```python
from build123d import *

# Parameters (mm, degrees)
BOSS_EXTRUDE1_DEPTH = 6.35


with BuildPart() as part:
    # Model → Boss-Extrude1 (new body)
    with BuildSketch(Plane.XY):
        with BuildLine():
            Line((-1e-09, 914.4), (-194.479849893, 914.4))
            ThreePointArc((-194.479849893, 914.4), (-204.918872942, 907.625287079), (-202.98320057, 895.332073104))
            ThreePointArc((-202.98320057, 895.332073104), (-164.535916974, 779.903104595), (-165.892020398, 658.247026365))
            Line((-165.892020398, 658.247026365), (-165.93888619, 658.129795087))
            ThreePointArc((-165.93888619, 658.129795087), (-191.627212467, 575.297388544), (-239.683438481, 503.105305724))
            ThreePointArc((-239.683438481, 503.105305724), (-421.799875665, 296.628923535), (-582.037423101, 72.747657041))
            ThreePointArc((-582.037423101, 72.747657041), (-620.33909224, 32.211350911), (-671.307126154, 9.573561873))
            ThreePointArc((-671.307126154, 9.573561873), (-674.990888605, 5.409489793), (-676.274252254, 0))
            ThreePointArc((-676.274252254, 0), (-674.990888605, -5.409489793), (-671.307126154, -9.573561873))
            ThreePointArc((-671.307126154, -9.573561873), (-620.33909224, -32.211350911), (-582.037423101, -72.747657041))
            ThreePointArc((-582.037423101, -72.747657041), (-421.799875665, -296.628923535), (-239.683438481, -503.105305724))
            ThreePointArc((-239.683438481, -503.105305724), (-191.627212467, -575.297388544), (-165.93888619, -658.129795087))
            Line((-165.93888619, -658.129795087), (-165.892020398, -658.247026365))
            ThreePointArc((-165.892020398, -658.247026365), (-164.535916974, -779.903104595), (-202.98320057, -895.332073104))
            ThreePointArc((-202.98320057, -895.332073104), (-204.918872942, -907.625287079), (-194.479849893, -914.4))
            Line((-194.479849893, -914.4), (-1e-09, -914.4))
            Line((-1e-09, -914.4), (194.47984989, -914.4))
            ThreePointArc((194.47984989, -914.4), (204.918872939, -907.625287079), (202.983200567, -895.332073104))
            ThreePointArc((202.983200567, -895.332073104), (164.535916972, -779.903104595), (165.892020395, -658.247026365))
            Line((165.892020395, -658.247026365), (165.938886187, -658.129795086))
            ThreePointArc((165.938886187, -658.129795086), (191.627212464, -575.297388544), (239.683438478, -503.105305724))
            ThreePointArc((239.683438478, -503.105305724), (421.79987566, -296.628923537), (582.037423094, -72.747657046))
            ThreePointArc((582.037423094, -72.747657046), (620.339092235, -32.211350913), (671.307126151, -9.573561873))
            ThreePointArc((671.307126151, -9.573561873), (674.990888602, -5.409489793), (676.274252251, 0))
            ThreePointArc((676.274252251, 0), (674.990888602, 5.409489793), (671.307126151, 9.573561873))
            ThreePointArc((671.307126151, 9.573561873), (620.339092237, 32.211350911), (582.037423097, 72.747657043))
            ThreePointArc((582.037423097, 72.747657043), (421.799875662, 296.628923535), (239.683438478, 503.105305724))
            ThreePointArc((239.683438478, 503.105305724), (191.627212464, 575.297388544), (165.938886187, 658.129795087))
            Line((165.938886187, 658.129795087), (165.892020395, 658.247026365))
            ThreePointArc((165.892020395, 658.247026365), (164.535916972, 779.903104595), (202.983200567, 895.332073104))
            ThreePointArc((202.983200567, 895.332073104), (204.918872939, 907.625287079), (194.47984989, 914.4))
            Line((194.47984989, 914.4), (-1e-09, 914.4))
        make_face()
        with BuildLine():
            Line((-46.0375, -761.999999999), (-46.0375, -609.361109078))
            ThreePointArc((-46.0375, -609.361109078), (-58.756065659, -548.411483153), (-94.788902893, -497.634978214))
            ThreePointArc((-94.788902893, -497.634978214), (-212.726110253, -352.63455945), (-285.980677563, -180.680860187))
            ThreePointArc((-285.980677563, -180.680860187), (-292.839641189, -146.846450496), (-298.006194276, -112.712605264))
            ThreePointArc((-298.006194276, -112.712605264), (-323.20694899, -65.087535088), (-373.608551252, -46.0375))
            Line((-373.608551252, -46.0375), (-457.356144829, -46.0375))
            ThreePointArc((-457.356144829, -46.0375), (-503.393644829, 0), (-457.356144829, 46.0375))
            Line((-457.356144829, 46.0375), (-373.608551252, 46.0375))
            ThreePointArc((-373.608551252, 46.0375), (-323.20694899, 65.087535088), (-298.006194276, 112.712605264))
            ThreePointArc((-298.006194276, 112.712605264), (-292.839641189, 146.846450496), (-285.980677563, 180.680860188))
            ThreePointArc((-285.980677563, 180.680860188), (-212.726110253, 352.63455945), (-94.788902893, 497.634978214))
            ThreePointArc((-94.788902893, 497.634978214), (-58.756065659, 548.411483153), (-46.0375, 609.361109078))
            Line((-46.0375, 609.361109078), (-46.0375, 761.999999999))
            ThreePointArc((-46.0375, 761.999999999), (0, 808.037499999), (46.0375, 761.999999999))
            Line((46.0375, 761.999999999), (46.0375, 609.361109078))
            ThreePointArc((46.0375, 609.361109078), (58.756065659, 548.411483153), (94.788902893, 497.634978214))
            ThreePointArc((94.788902893, 497.634978214), (212.726110253, 352.63455945), (285.980677563, 180.680860188))
            ThreePointArc((285.980677563, 180.680860188), (292.839641189, 146.846450496), (298.006194276, 112.712605264))
            ThreePointArc((298.006194276, 112.712605264), (323.20694899, 65.087535088), (373.608551252, 46.0375))
            Line((373.608551252, 46.0375), (457.356144829, 46.0375))
            ThreePointArc((457.356144829, 46.0375), (503.393644829, 0), (457.356144829, -46.0375))
            Line((457.356144829, -46.0375), (373.608551252, -46.0375))
            ThreePointArc((373.608551252, -46.0375), (323.20694899, -65.087535088), (298.006194276, -112.712605264))
            ThreePointArc((298.006194276, -112.712605264), (292.839641189, -146.846450497), (285.980677563, -180.680860188))
            ThreePointArc((285.980677563, -180.680860188), (212.726110253, -352.63455945), (94.788902893, -497.634978214))
            ThreePointArc((94.788902893, -497.634978214), (58.756065659, -548.411483153), (46.0375, -609.361109078))
            Line((46.0375, -609.361109078), (46.0375, -761.999999999))
            ThreePointArc((46.0375, -761.999999999), (0, -808.037499999), (-46.0375, -761.999999999))
        make_face(mode=Mode.SUBTRACT)
    extrude(amount=BOSS_EXTRUDE1_DEPTH)


solid = part.part
```
Geometry: final body of the model. Coordinates: model frame, mm. A direction names the side the tool comes from. Coordinates: 2 decimals unless noted, no trailing zeros. Order: outer loops, then holes, each group sorted by start corner. A loop starts at its lowest first (then second) coordinate and runs counter-clockwise, first axis right, second up. Notation, with made-up numbers: (72, 17.5) - (101, 17.5) arc R15 cw to (101, 40.5) - close; hole circle Ø5 at (79.5, -22). An arc over 180 degrees is marked (long way). Write each question's results on one line, items separated by ' | '.
1) Line query: line 1 (Y direction, x = -189.5, z = 3); line 2 (Y direction, x = -24.5, z = 4.5); line 3 (X direction, y = 295, z = 5). Output: solid intervals per line, ascending. Write a range as from..to.
Results list:
line 1: -914.4..-867.08, -579.87..-388.5, 388.5..579.87, 867.08..914.4 | line 2: -914.4..-800.98, 800.98..914.4 | line 3: -423.09..-243.76, 243.76..423.09
2) Pull-direction query (Y, two-part tool) for faces 1 (the cylindrical face through (419.4, -299.64, 3.13)), 2 (the flat face through (-304, -131, 6.35)), 3 (the cylindrical face through (214.08, -350.38, 3.13)); classes: pulls with the +Y half, pulls with the -Y half, needs draft (parallel to the pull), parting line crosses it, or undercut.
Results list:
face 1: pulls with the -Y half | face 2: needs draft | face 3: undercut
3) Section B-B, the plane y = 636. Return loops of the section in (x, z).
Results list:
outline: (-170.3, 0) - (-46.04, 0) - (-46.04, 6.35) - (-170.3, 6.35) - close; (46.04, 0) - (170.3, 0) - (170.3, 6.35) - (46.04, 6.35) - close
4) Section A-A, the plane x = 0. Return loops of the section in (y, z), plus the area to 3 significant figures.
Results list:
outline: (-914.4, 0) - (-808.04, 0) - (-808.04, 6.35) - (-914.4, 6.35) - close; (808.04, 0) - (914.4, 0) - (914.4, 6.35) - (808.04, 6.35) - close | area: 1,350 mm^2
5) Pin query (flat end, axial travel): pin 1 (1.9 mm diameter, centred on x = -410, z = 2, fed in from -Y); pin 2 (1 mm diameter, centred on y = -333.5, z = 4.5, fed in from +X); pin 3 (3 mm diameter, centred on x = -412, z = 4, fed in from +Y). Return the tip coordinate at first contact, or that it passes through.
Results list:
pin 1: y = -312.53 | pin 2: x = 392.35 | pin 3: y = 310.74
6) Set-up query: faces 4 (the cylindrical face through (-214.08, 350.38, 3.13)), 5 (the cylindrical face through (-192.15, -574.2, 3.13)), 6 (the cylindrical face through (424.2, 293.61, 3.13)). Return all of +Z, -Z, +X, -X, +Y, -Y with unobstructed straight access to the full face (end or side cutting, diameter ignored); none if empty.
Results list:
face 4: +Z, -Z | face 5: +Z, -Z, -X | face 6: +Z, -Z, +X, +Y
